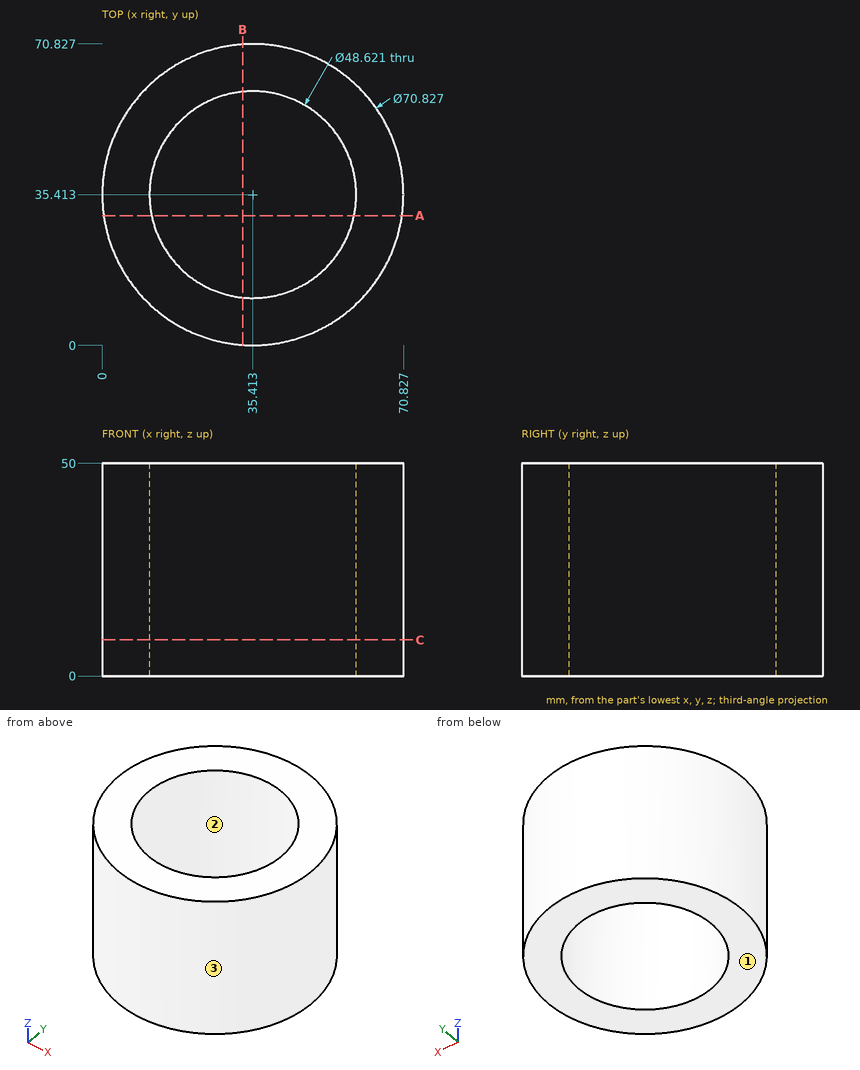
Part print with two shaded views. Sizes in mm from the minimum x, y, z corner. Give positions to 0.01 mm unless a question says otherwise; leave off trailing zeros. Order: outer loops, then holes, each group sorted by start corner. A loop starts at its lowest first (then second) coordinate and runs counter-clockwise, first axis right, second up.
1) Saw through at B-B, the plane x = 33. Write the cut outline in (y, z) (1 decimal).
2) Saw through at A-A, the plane y = 30.5. Write the cut outline in (x, z) (1 decimal).
3) Wall check: probe 1 along Y at (x, z) = (42, 14) (1 decimal); probe 2 along X at (y, z) = (16.5, 7) (1 decimal); probe 3 along X at (y, z) = (33, 31.5) (1 decimal). Give the ranges that are in metal, low to high.
4) Saw through at C-C, the plane z = 8.5. Write the cut outline in (x, y).
5) Pin check, flat tips, straight feed: pin 1 (12 mm diameter, centred on y = 58.5, z = 23, fed in from +X); pin 2 (2 mm diameter, centred on x = 49, z = 39.5, fed in from +Y) (1 decimal); pin 3 (8 mm diameter, centred on x = 7.5, z = 36.5, fed in from +Y) (1 decimal); pin 4 (12 mm diameter, centred on x = 45, y = 62.5, fed in from -Z). Stop position of each tip, or through.
6) Mould opens along X. For the marked faces 1, 2 and 3 say: +X half, -X half, draft (parallel to the pull), parting line (faces both ways), or undercut.
Computed:
1. outline: (0.1, 0) - (11.2, 0) - (11.2, 50) - (0.1, 50) - close; (59.6, 0) - (70.7, 0) - (70.7, 50) - (59.6, 50) - close
2. outline: (0.3, 0) - (11.6, 0) - (11.6, 50) - (0.3, 50) - close; (59.2, 0) - (70.5, 0) - (70.5, 50) - (59.2, 50) - close
3. probe 1: y = 0.6 to 12, 58.8 to 70.2
3. probe 2: x = 5.5 to 20.1, 50.7 to 65.4
3. probe 3: x = 0.1 to 11.2, 59.6 to 70.7
4. outline: circle Ø70.83 at (35.41, 35.41); hole circle Ø48.62 at (35.41, 35.41)
5. pin 1: stops at x = 66.43
5. pin 2: stops at y = 68.5
5. pin 3: stops at y = 61.5
5. pin 4: stops at z = 0
6. face 1: draft
6. face 2: undercut
6. face 3: parting line
